Source: CAD feature listing. Evaluate the final solid. Frame: model axes, mm. Give positions to 0.01 mm unless a question says otherwise; leave off trailing zeros. Write each loop counter-clockwise with the first axis right and the second up, starting at its lowest first coordinate (ties: lowest second). Pieces come first, ordered by that corner, then holes. Notation, with made-up numbers: M 87,-38 L 116,-38 A16 ccw 116,-19 Z; hole C 80,10.5 d2. An arc over 180 degrees is marked long. Return JSON: item names as keys, results as strings.
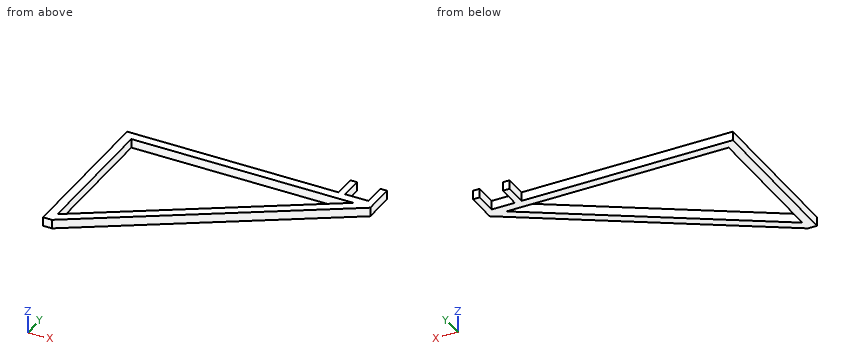
Autodesk Fusion 360 part; units mm, degrees
sketch "Sketch1" plane through (0, 0, 0) normal (0, 0, 1) x (1, 0, 0)
  line L0 (0, 0) -> (7.62, 0)
  line L1 (7.62, 0) -> (7.62, 134.62)
  line L2 (7.62, 134.62) -> (0, 134.62)
  line L3 (0, 134.62) -> (0, 0)
  line L4 (7.62, 134.62) -> (210.82, 134.62)
  line L5 (210.82, 134.62) -> (210.82, 127)
  line L6 (210.82, 127) -> (7.62, 127)
  line L7 (7.62, 127) -> (7.62, 134.62)
  line L8 (210.82, 127) -> (7.62, 0)
  line L9 (7.62, 0) -> (3.5814, 6.4617)
  line L10 (3.5814, 6.4617) -> (206.7814, 133.4617)
  line L11 (206.7814, 133.4617) -> (210.82, 127)
  line L12 (210.82, 134.62) -> (205.105, 134.62)
  line L13 (205.105, 134.62) -> (205.105, 153.67)
  line L14 (205.105, 153.67) -> (210.82, 153.67)
  line L15 (210.82, 153.67) -> (210.82, 134.62)
  line L16 (185.42, 134.62) -> (179.705, 134.62)
  line L17 (179.705, 134.62) -> (179.705, 153.6683)
  line L18 (179.705, 153.6683) -> (185.42, 153.6683)
  line L19 (185.42, 153.6683) -> (185.42, 134.62)
  dimension "d1" = 134.62
  dimension "d2" = 7.62
  dimension "d3" = 203.2
  dimension "d4" = 7.62
  dimension "d5" = 5.715
  dimension "d6" = 19.05
  dimension "d7" = 19.0483
  dimension "d8" = 5.715
extrude "Extrude1" add sketch "Sketch1" along normal blind 7.62 contours L0 L1 L2 L3 L7 L9 L10 | L1 L9 L10 | L1 L6 L8 L10 | L1 L4 L5 L6 L7 L10 L11 L12 L16 | L6 L10 L11 | L4 L12 L13 L14 L15 | L4 L16 L17 L18 L19
1) Contact query for flat-ended pins moving along their axis: pin 1 Ø4 at (x, z) = (191, 5) entering from +Y; pin 2 Ø4 at (y, z) = (141, 4.5) entering from -X (3 decimals); pin 3 Ø1.5 at (x, z) = (152, 1) entering from -Y; pin 4 Ø10 at (x, y) = (132, 80.5) entering from -Z. Output: stop coordinate, or through.
Numbers:
{"pin 1": "stops at y = 134.62", "pin 2": "stops at x = 179.705", "pin 3": "stops at y = 89.77", "pin 4": "stops at z = 0"}
2) Cut plane A-A, the plane y = 143.5. Return the cut outline in (x, z) (3 decimals), then the cut area to 3 significant figures.
Numbers:
{"outline": "M 179.705,0 L 185.42,0 L 185.42,7.62 L 179.705,7.62 Z; M 205.105,0 L 210.82,0 L 210.82,7.62 L 205.105,7.62 Z", "area": "87.1 mm²"}
3) Line query: line 1 (X direction, y = 140, z = 1.5) (3 decimals); line 2 (Y direction, x = 151, z = 1.25); line 3 (Y direction, x = 105, z = 6.5). Output: solid intervals per line, ascending. Write a range as [from, to].
Numbers:
{"line 1": "x = [179.705, 185.42], [205.105, 210.82]", "line 2": "y = [89.61, 98.6], [127, 134.62]", "line 3": "y = [60.86, 69.85], [127, 134.62]"}
4) Cut plane C-C, the plane z = 4.75. Return the cut outline in (x, y) (3 decimals).
Numbers:
{"outline": "M 0,0 L 7.62,0 L 210.82,127 L 210.82,153.67 L 205.105,153.67 L 205.105,134.62 L 185.42,134.62 L 185.42,153.668 L 179.705,153.668 L 179.705,134.62 L 0,134.62 Z; hole M 7.62,8.986 L 196.443,127 L 7.62,127 Z"}
5) Cut plane B-B, the plane x = 17.5. Return the cut outline in (y, z) (3 decimals).
Numbers:
{"outline": "M 6.175,0 L 15.161,0 L 15.161,7.62 L 6.175,7.62 Z; M 127,0 L 134.62,0 L 134.62,7.62 L 127,7.62 Z"}
